```python
from build123d import *

# Parameters (mm, degrees)
BOSS_EXTRUDE1_DEPTH   = 25.4
SKETCH2_R             = 2.75
CUT_EXTRUDE1_DEPTH    = 45.22263278
SKETCH3_R             = 4.500000017
CUT_EXTRUDE2_DEPTH    = 37.650283508
F_2_0MM_DOWEL_HOLE1_D = 2.1


with BuildPart() as part:
    # Sketch1 → Boss-Extrude1 (new body)
    with BuildSketch(Plane.XY):
        Polygon((-11.1125, 0), (11.1125, 0), (11.1125, 22.225), (14.2875, 22.225), (14.2875, -3.175), (-14.2875, -3.175), (-14.2875, 22.225), (-11.1125, 22.225), align=None)
    extrude(amount=BOSS_EXTRUDE1_DEPTH)

    # Sketch2 → Cut-Extrude1 (cut, through all)
    with BuildSketch(Plane(origin=(14.2875, 0, 0), x_dir=(0, 0, -1), z_dir=(1, 0, 0))):
        with Locations(Location((-12.7, 15.875, 0), (0, 0, 90))):
            Circle(SKETCH2_R)
        with Locations(Location((-12.7, 4.7625, 0), (0, 0, 90))):
            Circle(SKETCH2_R)
    extrude(amount=-CUT_EXTRUDE1_DEPTH, mode=Mode.SUBTRACT)

    # Sketch3 → Cut-Extrude2 (cut, through all)
    with BuildSketch(Plane(origin=(0, 0, 0), x_dir=(1, 0, 0), z_dir=(0, 1, 0))):
        with Locations(Location((0, -12.7, 0), (0, 0, 180))):
            Circle(SKETCH3_R)
    extrude(amount=-CUT_EXTRUDE2_DEPTH, mode=Mode.SUBTRACT)

    # Ø2.0mm Dowel Hole1 (through all)
    with Locations(Plane(origin=(0, 0, 0), x_dir=(1, 0, 0), z_dir=(0, 1, 0))):
        with Locations((0, -4.699999998), (5.656854251, -7.043145749), (8.000000002, -12.7), (5.656854251, -18.356854251), (0, -20.700000002), (-5.656854251, -18.356854251), (-8.000000002, -12.7), (-5.656854251, -7.043145749)):
            Hole(F_2_0MM_DOWEL_HOLE1_D / 2)


solid = part.part
```
The listing builds one solid part. Answer for the finished solid, in the listing's coordinates (mm). A direction names the side the tool comes from. Coordinates: 2 decimals unless noted, no trailing zeros. Order: outer loops, then holes, each group sorted by start corner. A loop starts at its lowest first (then second) coordinate and runs counter-clockwise, first axis right, second up. Notation, with made-up numbers: M 14,46 L 29,46 A23 ccw 29,65 Z; hole C 3,18 d2. An arc over 180 degrees is marked long. Answer as a JSON object with one key per item and string values. Group by question number.
1. A flat-ended cylindrical pin translates along its axis: P1, Ø2.5, axis at x = 5.66, z = 7.04, coming from the +Y side. Find the tip coordinate at first contact, or state that the pin passes through.
2. Section D-D on y = 3.5 is taken. Write down the section's boundary in (x, z), then the cut area to 3 significant figures.
3. Section B-B on x = 8 is taken. Write down the section's boundary in (y, z) (3 decimals).
4. Section A-A on y = 0.75 is taken. Write down the section's boundary in (x, z).
5. A tool of negligible diameter and unlimited length cuts with its end or side. For faces 1 (the flat face through (5, 0, 13)), 2 (the cylindrical face through (0.59, -1.57, 17.16)), from which of +Z, -Z, +X, -X, +Y, -Y can it reach the whole face along a straight path? Write none if from no direction.
6. Straight lines are drawn through the part: line 1 (X direction, y = 5, z = 22.5); line 2 (Y direction, x = -12, z = 11.5) (3 decimals); line 3 (Y direction, x = 10.25, z = 23.25) (3 decimals). For each, find the intervals that lie inside material, in ascending order.
7. Determine the mould class of faces 3 (the flat face through (11.112, 11, 13)), 4 (the cylindrical face through (12.72, 13.85, 14.56)), 5 (the flat face through (0, -1, 25.4)) for opening direction Z: released by +Z, released by -Z, zero draft, split by the parting line, or undercut.
Values follow:
{
 "1": {"P1": "y = 0"},
 "2": {"outline": "M -14.29,0 L -11.11,0 L -11.11,10.26 L -14.29,10.26 Z; M -14.29,15.14 L -11.11,15.14 L -11.11,25.4 L -14.29,25.4 Z; M 11.11,0 L 14.29,0 L 14.29,10.26 L 11.11,10.26 Z; M 11.11,15.14 L 14.29,15.14 L 14.29,25.4 L 11.11,25.4 Z", "area": "130 mm2"},
 "3": {"outline": "M -3.175,0 L 0,0 L 0,11.65 L -3.175,11.65 Z; M -3.175,13.75 L 0,13.75 L 0,25.4 L -3.175,25.4 Z"},
 "4": {"outline": "M -14.29,0 L -11.11,0 L -11.11,25.4 L -14.29,25.4 Z; M 11.11,0 L 14.29,0 L 14.29,25.4 L 11.11,25.4 Z"},
 "5": {"face 1": "+Z, -Z, +Y", "face 2": "+Y, -Y"},
 "6": {"line 1": "-14.29 to -11.11, 11.11 to 14.29", "line 2": "-3.175 to 2.288, 7.237 to 13.401, 18.349 to 22.225", "line 3": "-3.175 to 0"},
 "7": {"face 3": "zero draft", "face 4": "undercut", "face 5": "released by +Z"}
}
